CAD build for the part. Positions are in the model's coordinates, mm. Face numbers are marked on the shaded views. Give positions to 0.01 mm unless a question says otherwise; leave off trailing zeros. Loops run counter-clockwise (first coordinate to the right, second up) from the corner with the lowest first, then second, coordinate; pieces in that order, holes last. Notation, with made-up numbers: M 40.25,22.25 L 66.25,22.25 A16 ccw 66.25,44.25 Z; hole C 33,55.5 d7. An arc over 180 degrees is marked long. Answer as CSV lines item,"result".
from build123d import *

# Parameters (mm, degrees)
CROQUIS1_R              = 5.75
SALIENTE_EXTRUIR1_DEPTH = 56
CROQUIS2_R              = 4.15
CORTAR_EXTRUIR1_DEPTH   = 59.333566666
CHAFL_N1_SIZE           = 0.4
CHAFL_N2_SIZE           = 0.4


with BuildPart() as part:
    # Croquis1 → Saliente-Extruir1 (new body)
    with BuildSketch(Plane(origin=(0, 0, 0), x_dir=(-1, 0, 0), z_dir=(0, 0, -1))):
        with Locations((-5.8, 5.8)):
            Circle(CROQUIS1_R)
    extrude(amount=-SALIENTE_EXTRUIR1_DEPTH)

    # Croquis2 → Cortar-Extruir1 (cut, through all)
    with BuildSketch(Plane.XY.offset(56)):
        with Locations((5.8, 5.8)):
            Circle(CROQUIS2_R)
    extrude(amount=-CORTAR_EXTRUIR1_DEPTH, mode=Mode.SUBTRACT)

    # Chaflán1
    chafl_n1_edges = [part.edges().sort_by_distance(p)[0] for p in [
        (11.55, 5.8, 0),
    ]]
    chamfer(chafl_n1_edges, length=CHAFL_N1_SIZE)

    # Chaflán2
    chafl_n2_edges = [part.edges().sort_by_distance(p)[0] for p in [
        (11.55, 5.8, 56),
    ]]
    chamfer(chafl_n2_edges, length=CHAFL_N2_SIZE)


solid = part.part
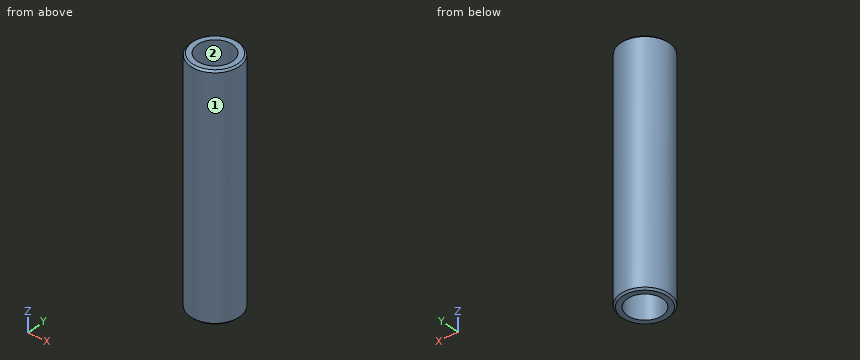
1) Band-saw the part on A-A on x = 5.8. Give the cut face in (y, z), and give its area (3 significant figures).
Answer below:
outline,"M 0.05,0.4 L 0.45,0 L 1.65,0 L 1.65,56 L 0.45,56 L 0.05,55.6 Z; M 9.95,0 L 11.15,0 L 11.55,0.4 L 11.55,55.6 L 11.15,56 L 9.95,56 Z"
area,"179 mm^2"
2) Flat gauge pins, fed straight in: pin 1 (1.5 mm diameter, centred on y = 8, z = 28, fed in from +X); pin 2 (3 mm diameter, centred on y = 9.5, z = 17.5, fed in from +X); pin 3 (3 mm diameter, centred on y = 10.5, z = 21.5, fed in from +X). Where does each tip first touch, or does it go through?
Answer below:
pin 1,"stops at x = 11.36"
pin 2,"stops at x = 11.11"
pin 3,"stops at x = 10.58"
3) Band-saw the part on C-C on z = 13. Give the cut face in (x, y), and give its area (3 significant figures).
Answer below:
outline,"C 5.8,5.8 d11.5; hole C 5.8,5.8 d8.3"
area,"49.8 mm^2"
4) Drill centre lines: line 1 (Y direction, x = 5.8, z = 15); line 2 (Y direction, x = 3.5, z = 24.5). Where is each one in solid material? Low to high. Write a range as from..to.
Answer below:
line 1,"y = 0.05..1.65, 9.95..11.55"
line 2,"y = 0.53..2.35, 9.25..11.07"
5) Mould opens along X. For the marked faces 1 and 2 say: +X half, -X half, draft (parallel to the pull), parting line (faces both ways), or undercut.
Answer below:
face 1,"parting line"
face 2,"undercut"
